from build123d import *

# Parameters (mm, degrees)
BOSS_EXTRUDE2_DEPTH = 1.5875
FILLET2_R           = 1


with BuildPart() as part:
    # Sketch1 → Boss-Extrude2 (new, symmetric)
    with BuildSketch(Plane.XY):
        with BuildLine():
            Line((-6.5, -1.935), (-6.5, -3.702326971))
            ThreePointArc((-6.5, -3.702326971), (-6.004381337, -3.801687055), (-5.5, -3.835))
            Line((-5.5, -3.835), (5.5, -3.835))
            ThreePointArc((5.5, -3.835), (6.004381337, -3.801687055), (6.5, -3.702326971))
            Line((6.5, -3.702326971), (6.5, -1.935))
            Line((6.5, -1.935), (6.5, 1.935))
            Line((6.5, 1.935), (6.5, 3.702326971))
            ThreePointArc((6.5, 3.702326971), (6.004381337, 3.801687055), (5.5, 3.835))
            Line((5.5, 3.835), (-5.5, 3.835))
            ThreePointArc((-5.5, 3.835), (-6.004381337, 3.801687055), (-6.5, 3.702326971))
            Line((-6.5, 3.702326971), (-6.5, 1.935))
            Line((-6.5, 1.935), (-6.5, -1.935))
        make_face()
        with BuildLine():
            Line((-5.5, 2.835), (-5.5, 1.935))
            ThreePointArc((-5.5, 1.935), (-3.565, 0), (-5.5, -1.935))
            Line((-5.5, -1.935), (-5.5, -2.835))
            ThreePointArc((-5.5, -2.835), (-2.665, 0), (-5.5, 2.835))
        make_face(mode=Mode.SUBTRACT)
        with BuildLine():
            Line((5.5, -1.935), (5.5, -2.835))
            ThreePointArc((5.5, -2.835), (2.665, 0), (5.5, 2.835))
            Line((5.5, 2.835), (5.5, 1.935))
            ThreePointArc((5.5, 1.935), (3.565, 0), (5.5, -1.935))
        make_face(mode=Mode.SUBTRACT)
    extrude(amount=BOSS_EXTRUDE2_DEPTH, both=True)

    # Fillet2
    fillet2_edges = [part.edges().sort_by_distance(p)[0] for p in [
        (6.5, -3.702326971, 0),
        (-6.5, -3.702326971, 0),
        (6.5, 3.702326971, 0),
        (-6.5, 3.702326971, 0),
    ]]
    fillet(fillet2_edges, radius=FILLET2_R - 0.0001)  # a hair under: the kernel refuses the full size


solid = part.part
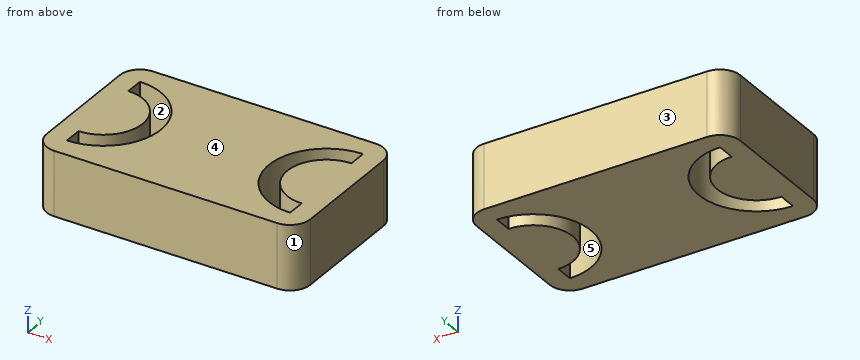
Can you work these out from the model? Positions are in its coordinate system, mm. Face numbers are marked on the shaded views. A direction names the side the tool comes from. Give positions to 0.01 mm unless a question says otherwise; leave off trailing zeros. Loops run counter-clockwise (first coordinate to the right, second up) from the corner with the lowest first, then second, coordinate; pieces in that order, holes last. Notation, with made-up numbers: (2, -23.5) - (44, -23.5) arc R16 ccw to (44, -9.5) - close; hole circle Ø4 at (49.25, 73.25). An arc over 180 degrees is marked (long way). Answer as a JSON object with one key per item and string values.
Q1. Imagine slicing it at A-A on z = -1. Give the number of separate pieces and of enclosed holes in the cut face, plus the area to 3 significant figures.
Geometry says:
{"separate pieces": "1", "enclosed holes": "2", "area": "85.4 mm²"}
Q2. Which directions (+Z, -Z, +X, -X, +Y, -Y) give clear straight access to the entire face, cutting with the end or side of a thin tool? Please do the marked faces 1 and 2.
Geometry says:
{"face 1": "+Z, -Z, +X, -Y", "face 2": "+Z, -Z"}
Q3. Imagine slicing it at B-B on y = 0. Write out the boundary of the cut face in (x, z) (1 decimal).
Geometry says:
{"outline": "(-6.5, -1.6) - (-3.6, -1.6) - (-3.6, 1.6) - (-6.5, 1.6) - close; (-2.7, -1.6) - (2.7, -1.6) - (2.7, 1.6) - (-2.7, 1.6) - close; (3.6, -1.6) - (6.5, -1.6) - (6.5, 1.6) - (3.6, 1.6) - close"}
Q4. Imagine slicing it at C-C on y = -1.25. Write out the boundary of the cut face in (x, z), plus the area to 3 significant figures.
Geometry says:
{"outline": "(-6.5, -1.59) - (-4.02, -1.59) - (-4.02, 1.59) - (-6.5, 1.59) - close; (-2.96, -1.59) - (2.96, -1.59) - (2.96, 1.59) - (-2.96, 1.59) - close; (4.02, -1.59) - (6.5, -1.59) - (6.5, 1.59) - (4.02, 1.59) - close", "area": "34.5 mm²"}
Q5. If we mould it in two halves opening along Y, with no side actions, what happens to the marked faces 3, 4 and 5? For each: pulls with the +Y half, pulls with the -Y half, needs draft (parallel to the pull), parting line crosses it, or undercut.
Geometry says:
{"face 3": "pulls with the +Y half", "face 4": "needs draft", "face 5": "undercut"}
Q6. If I drill on L1, parallel to X at y = -1.25, z = 0.2; L2, parallel to X at y = -1.5, z = -0.3; L3, parallel to Y at x = -4.5, z = -0.6 (3 decimals), over which ranges is the centre line in solid material (lowest first)?
Geometry says:
{"L1": "-6.5 to -4.02, -2.96 to 2.96, 4.02 to 6.5", "L2": "-6.5 to -4.28, -3.09 to 3.09, 4.28 to 6.5", "L3": "-3.835 to -2.653, -1.657 to 1.657, 2.653 to 3.835"}
